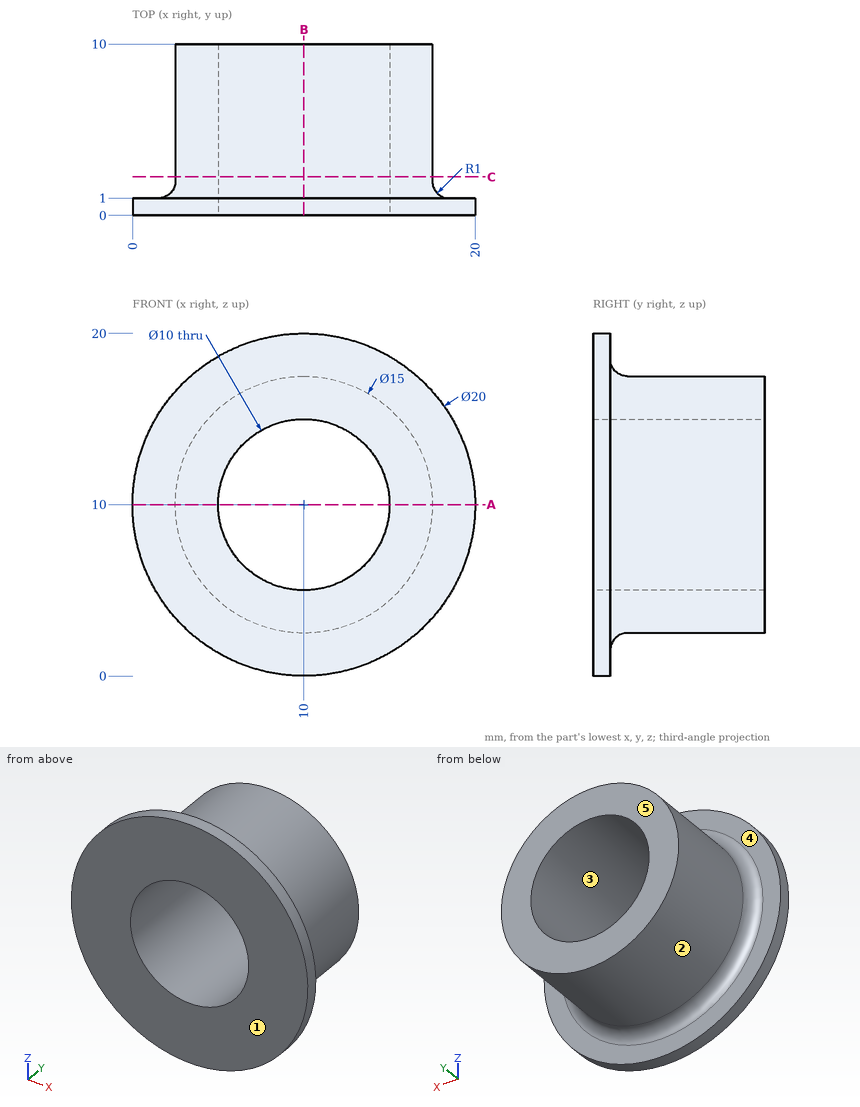
Design review of the part shown in the three views and the two pictorial views. Dimensions are in mm from the part's minimum x, y and z. A direction names the side the tool comes from. Round coordinates to 2 decimals unless told otherwise and drop trailing zeros. Write each loop counter-clockwise with the first axis right and the second up, starting at its lowest first coordinate (ties: lowest second). Pieces come first, ordered by that corner, then holes. Notation, with made-up numbers: M 62,35 L 91,35 A18 ccw 91,49 Z; hole C 6,47.25 d5. An arc over 180 degrees is marked long. Use a Markdown table: item, result. Add a question column.
Q1. To check wall thickness, follow line 1 (Z direction, x = 9.75, y = 8.25); line 2 (X direction, y = 5.5, z = 10); line 3 (Z direction, x = 14.5, y = 4). State the ranges of each line that lie inside material, in increasing order.
Q2. We need section B-B, the plane x = 10. State the section outline as (y, z) points, plus the area to 3 significant figures.
Q3. Insertion check: pin 1 (1 mm diameter, centred on x = 15, y = 5, fed in from -Z); pin 2 (2 mm diameter, centred on x = 9, y = 6, fed in from +Z); pin 3 (8 mm diameter, centred on x = 10, z = 10, fed in from -Y). Each pin has a flat end and moves straight along its axis. Give the tip position at first contact, or say it passes through.
Q4. We need section A-A, the plane z = 10. State the section outline as (x, y) points.
Q5. Machinability: for the marked faces 4 and 5, which of the approach directions +Z, -Z, +X, -X, +Y, -Y give a long, thin tool a straight path to every point of the face, cutting with its end or side? Answer none if there is none.
Q6. The part is to be moulded in two halves that separate along X. For the marked faces 1, 2 and 3, say which applies: pulls with the +X half, pulls with the -X half, needs draft (parallel to the pull), parting line crosses it, or undercut.
Q7. We need section C-C, the plane y = 2.25. State the section outline as (x, z) points.
Findings below:
| question | item | result |
|---|---|---|
| 1 | line 1 | z = 2.5 to 5.01, 14.99 to 17.5 |
| 1 | line 2 | x = 2.5 to 5, 15 to 17.5 |
| 1 | line 3 | z = 4 to 7.82, 12.18 to 16 |
| 2 | outline | M 0,0 L 1,0 L 1,1.5 A1 cw 2,2.5 L 10,2.5 L 10,5 L 0,5 Z; M 0,15 L 10,15 L 10,17.5 L 2,17.5 A1 cw 1,18.5 L 1,20 L 0,20 Z |
| 2 | area | 55.4 mm² |
| 3 | pin 1 | stops at z = 4 |
| 3 | pin 2 | stops at z = 17.5 |
| 3 | pin 3 | passes through |
| 4 | outline | M 0,0 L 5,0 L 5,10 L 2.5,10 L 2.5,2 A1 cw 1.5,1 L 0,1 Z; M 15,0 L 20,0 L 20,1 L 18.5,1 A1 cw 17.5,2 L 17.5,10 L 15,10 Z |
| 5 | face 4 | +Y |
| 5 | face 5 | +Z, -Z, +X, -X, +Y |
| 6 | face 1 | needs draft |
| 6 | face 2 | parting line crosses it |
| 6 | face 3 | undercut |
| 7 | outline | C 10,10 d15; hole C 10,10 d10 |
